Model file for the job. Use its own axes, mm. Face numbers are marked on the shaded views. A direction names the side the tool comes from. Coordinates: 2 decimals unless noted, no trailing zeros. Order: outer loops, then holes, each group sorted by start corner. A loop starts at its lowest first (then second) coordinate and runs counter-clockwise, first axis right, second up. Notation, with made-up numbers: (-30.75, 47.5) -> (10.25, 47.5) arc R29 cw to (10.25, 81.5) -> close; hole circle Ø10 at (30, 4.25). An arc over 180 degrees is marked (long way). Use CSV: the item, a comma, the result in double quotes. Start each with the question number.
(1) Pin check, flat tips, straight feed: pin 1 Ø2.5 at (x, y) = (30.11, 15) entering from +Z; pin 2 Ø5 at (y, z) = (4.5, 5) entering from +X. Stop position of each tip, or through.
(2) Tool access for the marked faces 1 and 2: list every direction of +Z, -Z, +X, -X, +Y, -Y with a clear straight run to the whole face (end or side of a thin tool).
(3) Cut at B-B on x = -7.5. Write the cut outline in (y, z).
(4) Cut at A-A on y = 15. Write the cut outline in (x, z).
(5) Cut at C-C on z = -5.5. Write the cut outline in (x, y).
(6) Cut at D-D on z = -11. Write the cut outline in (x, y), plus the area to 3 significant figures.
(7) Probe L1, parallel to Y at x = -17, z = 12; L2, parallel to X at y = 20.5, z = 10; L3, parallel to X at y = 27, z = -10. List the from-to ranges inside material, lowest first.
(8) Pull direction Z, two halves, no side cores. Call the marked faces 3, 4 and 5: pulls with the +Z half, pulls with the -Z half, needs draft (parallel to the pull), parting line crosses it, or undercut.
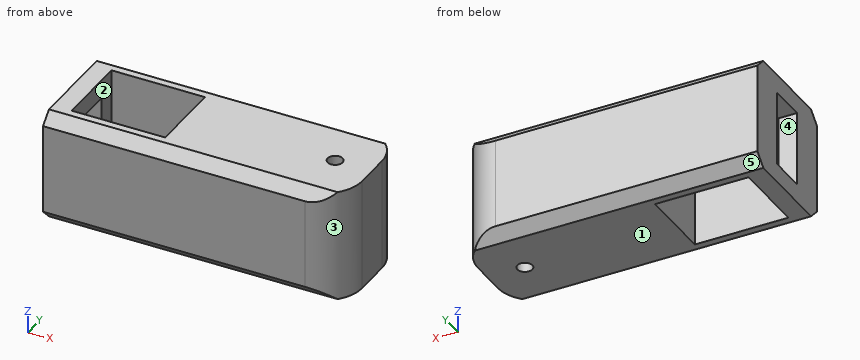
```python
from build123d import *

# Parameters (mm, degrees)
SKETCH1_W           = 80
SKETCH1_H           = 30
BOSS_EXTRUDE1_DEPTH = 30
SKETCH2_R           = 2
CUT_EXTRUDE1_DEPTH  = 30
CHAMFER1_SIZE       = 3
SKETCH3_W           = 25
SKETCH3_H           = 20
CUT_EXTRUDE2_DEPTH  = 30
SKETCH4_W           = 20
SKETCH4_H           = 10
CUT_EXTRUDE3_DEPTH  = 20
FILLET1_R           = 10


with BuildPart() as part:
    # Sketch1 → Boss-Extrude1 (new body)
    with BuildSketch(Plane(origin=(0, 0, 0), x_dir=(1, 0, 0), z_dir=(0, 1, 0))):
        Rectangle(SKETCH1_W, SKETCH1_H)
    extrude(amount=BOSS_EXTRUDE1_DEPTH)

    # Sketch2 → Cut-Extrude1 (cut)
    with BuildSketch(Plane.XY.offset(15)):
        with Locations((30.11486463, 15)):
            Circle(SKETCH2_R)
    extrude(amount=-CUT_EXTRUDE1_DEPTH, mode=Mode.SUBTRACT)

    # Chamfer1
    chamfer1_edges = [part.edges().sort_by_distance(p)[0] for p in [
        (0, 30, 15),
        (0, 0, 15),
        (0, 0, -15),
        (0, 30, -15),
    ]]
    chamfer(chamfer1_edges, length=CHAMFER1_SIZE)

    # Sketch3 → Cut-Extrude2 (cut)
    with BuildSketch(Plane(origin=(0, 0, -15), x_dir=(-1, 0, 0), z_dir=(0, 0, -1))):
        with Locations((22.5, 15)):
            Rectangle(SKETCH3_W, SKETCH3_H)
    extrude(amount=-CUT_EXTRUDE2_DEPTH, mode=Mode.SUBTRACT)

    # Sketch4 → Cut-Extrude3 (cut)
    with BuildSketch(Plane.ZY.offset(40)):
        with Locations((0, 15)):
            Rectangle(SKETCH4_W, SKETCH4_H)
    extrude(amount=-CUT_EXTRUDE3_DEPTH, mode=Mode.SUBTRACT)

    # Fillet1
    fillet1_edges = [part.edges().sort_by_distance(p)[0] for p in [
        (40, 0, 0),
        (40, 30, 0),
    ]]
    fillet(fillet1_edges, radius=FILLET1_R)


solid = part.part
```
Outcome:
1,pin 1,"through"
1,pin 2,"x = 39.54"
2,face 1,"-Z, +X, -X, +Y, -Y"
2,face 2,"+Z, -Z"
3,outline,"(0, -12) -> (3, -15) -> (27, -15) -> (30, -12) -> (30, 12) -> (27, 15) -> (3, 15) -> (0, 12) -> close"
4,outline,"(-40, -15) -> (-35, -15) -> (-35, -10) -> (-40, -10) -> close; (-40, 10) -> (-35, 10) -> (-35, 15) -> (-40, 15) -> close; (-10, -15) -> (28.11, -15) -> (28.11, 15) -> (-10, 15) -> close; (32.11, -15) -> (40, -15) -> (40, 15) -> (32.11, 15) -> close"
5,outline,"(-40, 0) -> (30, 0) arc R10 ccw to (40, 10) -> (40, 20) arc R10 ccw to (30, 30) -> (-40, 30) -> (-40, 20) -> (-35, 20) -> (-35, 25) -> (-10, 25) -> (-10, 5) -> (-35, 5) -> (-35, 10) -> (-40, 10) -> close; hole circle Ø4 at (30.11, 15)"
6,outline,"(-40, 0) -> (30, 0) arc R10 ccw to (40, 10) -> (40, 20) arc R10 ccw to (30, 30) -> (-40, 30) -> close; hole (-35, 5) -> (-10, 5) -> (-10, 25) -> (-35, 25) -> close; hole circle Ø4 at (30.11, 15)"
6,area,"1,840 mm2"
7,L1,"0 to 5, 25 to 30"
7,L2,"-40 to -35, -10 to 39.99"
7,L3,"-40 to 37.14"
8,face 3,"needs draft"
8,face 4,"undercut"
8,face 5,"pulls with the -Z half"
